```python
from build123d import *

# Parameters (mm, degrees)
BOSS_EXTRUDE1_DEPTH = 10
BOSS_EXTRUDE2_DEPTH = 70
SKETCH5_W           = 190
SKETCH5_H           = 80
CUT_EXTRUDE1_DEPTH  = 70
SKETCH6_R           = 7
CUT_EXTRUDE2_DEPTH  = 401.249921924


with BuildPart() as part:
    # Sketch2 → Boss-Extrude1 (new body)
    with BuildSketch(Plane(origin=(0, 0, 0), x_dir=(1, 0, 0), z_dir=(0, 1, 0))):
        with BuildLine():
            Line((-180, -130), (180, -130))
            ThreePointArc((180, -130), (183.535533906, -128.535533906), (185, -125))
            Line((185, -125), (185, 125))
            ThreePointArc((185, 125), (183.535533906, 128.535533906), (180, 130))
            Line((180, 130), (-180, 130))
            ThreePointArc((-180, 130), (-183.535533906, 128.535533906), (-185, 125))
            Line((-185, 125), (-185, -125))
            ThreePointArc((-185, -125), (-183.535533906, -128.535533906), (-180, -130))
        make_face()
    extrude(amount=BOSS_EXTRUDE1_DEPTH)

    # Sketch3 → Boss-Extrude2 (add)
    with BuildSketch(Plane(origin=(0, 10, 0), x_dir=(1, 0, 0), z_dir=(0, 1, 0))):
        with BuildLine():
            Line((180, 130), (-180, 130))
            ThreePointArc((-180, 130), (-183.535533906, 128.535533906), (-185, 125))
            Line((-185, 125), (-185, -125))
            ThreePointArc((-185, -125), (-183.535533906, -128.535533906), (-180, -130))
            Line((-180, -130), (180, -130))
            ThreePointArc((180, -130), (183.535533906, -128.535533906), (185, -125))
            Line((185, -125), (185, 125))
            ThreePointArc((185, 125), (183.535533906, 128.535533906), (180, 130))
        make_face()
        with BuildLine():
            Line((170, 120), (-170, 120))
            ThreePointArc((-170, 120), (-173.535533906, 118.535533906), (-175, 115))
            Line((-175, 115), (-175, -115))
            ThreePointArc((-175, -115), (-173.535533906, -118.535533906), (-170, -120))
            Line((-170, -120), (170, -120))
            ThreePointArc((170, -120), (173.535533906, -118.535533906), (175, -115))
            Line((175, -115), (175, 115))
            ThreePointArc((175, 115), (173.535533906, 118.535533906), (170, 120))
        make_face(mode=Mode.SUBTRACT)
    extrude(amount=BOSS_EXTRUDE2_DEPTH)

    # Sketch5 → Cut-Extrude1 (cut)
    with BuildSketch(Plane(origin=(0, 0, -130), x_dir=(-1, 0, 0), z_dir=(0, 0, -1))):
        with Locations((0, 80)):
            Rectangle(SKETCH5_W, SKETCH5_H)
    extrude(amount=-CUT_EXTRUDE1_DEPTH, mode=Mode.SUBTRACT)

    # Sketch6 → Cut-Extrude2 (cut, through all)
    with BuildSketch(Plane(origin=(185, 0, 0), x_dir=(0, 0, -1), z_dir=(1, 0, 0))):
        with Locations((0, 61)):
            Circle(SKETCH6_R)
    extrude(amount=-CUT_EXTRUDE2_DEPTH, mode=Mode.SUBTRACT)


solid = part.part
```
Here's how the part is built. I have some questions about the finished solid (model axes, mm). A direction names the side the tool comes from. Coordinates: 2 decimals unless noted, no trailing zeros. Write each loop counter-clockwise with the first axis right and the second up, starting at its lowest first coordinate (ties: lowest second). Pieces come first, ordered by that corner, then holes. Notation, with made-up numbers: (30, 47.5) -> (63, 47.5) arc R16 cw to (63, 63.5) -> close; hole circle Ø8 at (5.5, 67.5). An arc over 180 degrees is marked (long way). Use a Markdown table: item, result. Add a question column.
(1) If we section it at C-C, the plane x = -101: Write out the boundary of the cut face in (y, z), and give its area (3 significant figures).
(2) We'd pull the mould along X, two halves only. Please class faces 1 (the flat face through (185, 39, 2)), 2 (the flat face through (95, 60, -125)), 3 (the flat face through (-1, 80, 125)): +X half, -X half, draft (parallel to the pull), parting line (faces both ways), or undercut.
(3) If we section it at A-A, the plane y = 61: Write out the boundary of the cut face in (x, z).
(4) For faces 4 (the flat face through (2, 37, -120)), 5 (the flat face through (-185, 39, -2)), 6 (the flat face through (-95, 60, -125)), which set-ups out of +Z, -Z, +X, -X, +Y, -Y let a thin tool reach every point of the face, with its end or its side?
(5) If we section it at D-D, the plane z = 103: Write out the boundary of the cut face in (x, y), and give its area (3 significant figures).
(6) Please list where these lines run through material, in increasing order: line 1 (X direction, y = 39.5, z = -95); line 2 (Z direction, x = 15, y = 18.5); line 3 (Y direction, x = 182, z = 0).
(7) If we section it at B-B, the plane z = 0: Write out the boundary of the cut face in (x, y), and give its area (3 significant figures).
(8) I'm going to push flat-ended pins straight in: P1, Ø3, axis at x = 27, z = -123, coming from the +Y side; P2, Ø12, axis at x = 28.5, z = 46.5, coming from the +Y side. Where does each tip first touch, or does it pass through?
Outcome:
| question | item | result |
|---|---|---|
| 1 | outline | (0, -130) -> (80, -130) -> (80, -120) -> (10, -120) -> (10, 120) -> (80, 120) -> (80, 130) -> (0, 130) -> close |
| 1 | area | 4,000 mm^2 |
| 2 | face 1 | +X half |
| 2 | face 2 | undercut |
| 2 | face 3 | draft |
| 3 | outline | (-185, -125) arc R5 ccw to (-180, -130) -> (-95, -130) -> (-95, -120) -> (-170, -120) arc R5 cw to (-175, -115) -> (-175, -7) -> (-185, -7) -> close; (-185, 7) -> (-175, 7) -> (-175, 115) arc R5 cw to (-170, 120) -> (170, 120) arc R5 cw to (175, 115) -> (175, 7) -> (185, 7) -> (185, 125) arc R5 ccw to (180, 130) -> (-180, 130) arc R5 ccw to (-185, 125) -> close; (95, -130) -> (180, -130) arc R5 ccw to (185, -125) -> (185, -7) -> (175, -7) -> (175, -115) arc R5 cw to (170, -120) -> (95, -120) -> close |
| 4 | face 4 | +Y |
| 4 | face 5 | +Z, -Z, -X, +Y, -Y |
| 4 | face 6 | -Z, +Y |
| 5 | outline | (-185, 0) -> (185, 0) -> (185, 80) -> (175, 80) -> (175, 10) -> (-175, 10) -> (-175, 80) -> (-185, 80) -> close |
| 5 | area | 5,100 mm^2 |
| 6 | line 1 | x = -185 to -175, 175 to 185 |
| 6 | line 2 | z = -130 to -120, 120 to 130 |
| 6 | line 3 | y = 0 to 54, 68 to 80 |
| 7 | outline | (-185, 0) -> (185, 0) -> (185, 54) -> (175, 54) -> (175, 10) -> (-175, 10) -> (-175, 54) -> (-185, 54) -> close; (-185, 68) -> (-175, 68) -> (-175, 80) -> (-185, 80) -> close; (175, 68) -> (185, 68) -> (185, 80) -> (175, 80) -> close |
| 7 | area | 4,820 mm^2 |
| 8 | P1 | stops at y = 40 |
| 8 | P2 | stops at y = 10 |
